Geometry check sheet. Reference: drawing and pictorial views, mm from the part's lowest x, y, z. A direction names the side the tool comes from. Round coordinates to 2 decimals unless told otherwise and drop trailing zeros. Loops run counter-clockwise (first coordinate to the right, second up) from the corner with the lowest first, then second, coordinate; pieces in that order, holes last. Notation, with made-up numbers: (31, 10.5) -> (90, 10.5) arc R24 cw to (90, 44.5) -> close; hole circle Ø3 at (79.5, 75.25). An arc over 180 degrees is marked (long way). Write item = value, one per line.
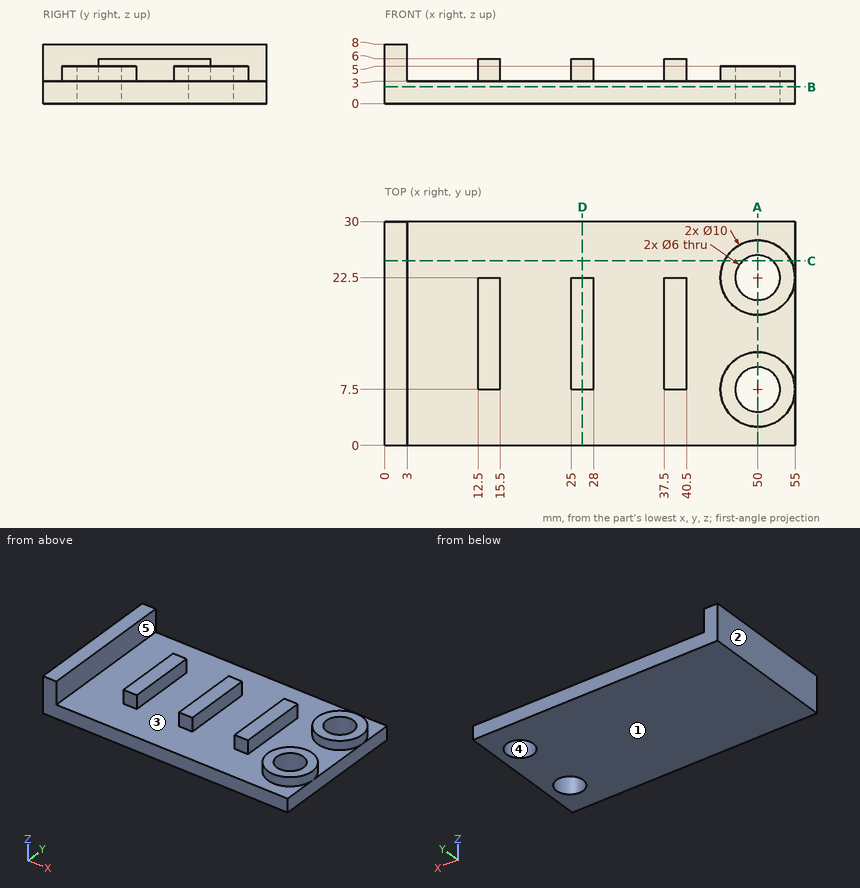
(1) Sectioned sample at B-B, the plane z = 2.25. Record the cut outline in (x, y), and give its area (3 significant figures).
Filled sheet:
outline = (0, 0) -> (55, 0) -> (55, 30) -> (0, 30) -> close; hole circle Ø6 at (50, 7.5); hole circle Ø6 at (50, 22.5)
area = 1,590 mm2
(2) Sectioned sample at D-D, the plane x = 26.5. Record the cut outline in (y, z).
Filled sheet:
outline = (0, 0) -> (30, 0) -> (30, 3) -> (22.5, 3) -> (22.5, 6) -> (7.5, 6) -> (7.5, 3) -> (0, 3) -> close
(3) Material ranges on probe 1 along Y at (x, z) = (50, 1.2); probe 2 along Y at (x, z) = (50, 3.8); probe 3 along Z at (x, y) = (5.5, 23.25), recorded low to high. Write a range as from..to.
Filled sheet:
probe_1 = 0..4.5, 10.5..19.5, 25.5..30
probe_2 = 2.5..4.5, 10.5..12.5, 17.5..19.5, 25.5..27.5
probe_3 = 0..3
(4) Draft check along X on the marked faces 1, 2 and 3. Enter one of: released by +X, released by -X, zero draft, split by the parting line, or undercut.
Filled sheet:
face_1 = zero draft
face_2 = released by -X
face_3 = undercut
(5) Set-up check for the marked faces 4 and 5: record each of +Z, -Z, +X, -X, +Y, -Y from which the full face is reachable in a straight line by a thin tool's end or side.
Filled sheet:
face_4 = +Z, -Z
face_5 = +Z, +Y, -Y
(6) Go/stop test with flat-tipped pins: pin 1 Ø1.5 at (y, z) = (12, 4.5) entering from +X; pin 2 Ø3.5 at (x, y) = (39, 16) entering from +Z; pin 3 Ø0.9 at (x, z) = (27, 4) entering from +Y. Record where each tip stops, or that it passes through.
Filled sheet:
pin_1 = 53.31
pin_2 = 6
pin_3 = 22.5
(7) Sectioned sample at C-C, the plane y = 24.75. Record the cut outline in (x, z).
Filled sheet:
outline = (0, 0) -> (48.02, 0) -> (48.02, 5) -> (45.53, 5) -> (45.53, 3) -> (3, 3) -> (3, 8) -> (0, 8) -> close; (51.98, 0) -> (55, 0) -> (55, 3) -> (54.47, 3) -> (54.47, 5) -> (51.98, 5) -> close
(8) Sectioned sample at A-A, the plane x = 50. Record the cut outline in (y, z).
Filled sheet:
outline = (0, 0) -> (4.5, 0) -> (4.5, 5) -> (2.5, 5) -> (2.5, 3) -> (0, 3) -> close; (10.5, 0) -> (19.5, 0) -> (19.5, 5) -> (17.5, 5) -> (17.5, 3) -> (12.5, 3) -> (12.5, 5) -> (10.5, 5) -> close; (25.5, 0) -> (30, 0) -> (30, 3) -> (27.5, 3) -> (27.5, 5) -> (25.5, 5) -> close
